For this review, take the finished solid that the model builds, in its own axes (mm). Face numbers are marked on the shaded views. A direction names the side the tool comes from. Coordinates: 2 decimals unless noted, no trailing zeros. Write each loop counter-clockwise with the first axis right and the second up, starting at its lowest first coordinate (ties: lowest second). Pieces come first, ordered by that corner, then holes. Notation, with made-up numbers: (88, -2.75) -> (105, -2.75) arc R19 cw to (105, 30.25) -> close; hole circle Ø4 at (-3, 24.5). An arc over 180 degrees is marked (long way). One line per item, written item: value. Start each with the question number.
1) Machinability: for the marked faces 4 and 5, which of the approach directions +Z, -Z, +X, -X, +Y, -Y give a long, thin tool a straight path to every point of the face, cutting with its end or side? Answer none if there is none.
2) Add section C-C (x = -0.6). State the section outline as (y, z) points, and give its area (3 significant figures).
3) Mouldability with a two-part tool opening along Z and no side actions: class the marked faces 1, 2 and 3 as released by +Z, released by -Z, zero draft, split by the parting line, or undercut.
4) Add section A-A (z = 0). State the section outline as (x, y) points, and give its area (3 significant figures).
5) For pin 1 Ø1.5 at (x, y) = (0, -2) entering from -Z; pin 2 Ø1 at (x, z) = (0.5, -2) entering from +Y; pin 3 Ø1.5 at (x, z) = (0, 1.5) entering from -Y, all flat-tipped, find the tip position at first contact; note any pin that passes through.
6) Add section D-D (x = 2.25). State the section outline as (y, z) points.
7) For probe 1 along Z at (x, y) = (0.2, 0); probe 2 along Z at (x, y) = (0.35, -0.65); probe 3 along X at (y, z) = (2.1, -0.2), list the stretches that pass through material, from the lowest coordinate up. Write a range as from..to.
from build123d import *

# Parameters (mm, degrees)
F0_R     = 2.85
F1_DEPTH = 3
F2_SIZE2 = 0.6
F2_SIZE  = 0.4
F3_R     = 1.45
F4_DEPTH = 2
F5_R     = 1.95
F5_R_2   = 1.45
F6_DEPTH = 0.5
F7_SIZE  = 0.2


with BuildPart() as f1:
    # F0 (on Right) → F1 (new body)
    with BuildSketch(Plane.YZ):
        Circle(F0_R)
    extrude(amount=F1_DEPTH)

    # F2
    f2_edges = [f1.edges().sort_by_distance(p)[0] for p in [
        (3, -2.85, 0),
    ]]
    f2_side = f1.faces().sort_by_distance((3, 0, 0))[0]
    chamfer(f2_edges, length=F2_SIZE, length2=F2_SIZE2, reference=f2_side)

    # F3 (on face) → F4 (join)
    with BuildSketch(Plane(origin=(0, 0, 0), x_dir=(0, -1, 0), z_dir=(-1, 0, 0))):
        Circle(F3_R)
    extrude(amount=F4_DEPTH)

    # F5 (on face) → F6 (cut)
    with BuildSketch(Plane(origin=(0, 0, 0), x_dir=(0, -1, 0), z_dir=(-1, 0, 0))):
        Circle(F5_R)
        Circle(F5_R_2, mode=Mode.SUBTRACT)
    extrude(amount=-F6_DEPTH, mode=Mode.SUBTRACT)

    # F7
    f7_edges = [f1.edges().sort_by_distance(p)[0] for p in [
        (0.5, 1.95, 0),
    ]]
    chamfer(f7_edges, length=F7_SIZE)


solid = f1.part
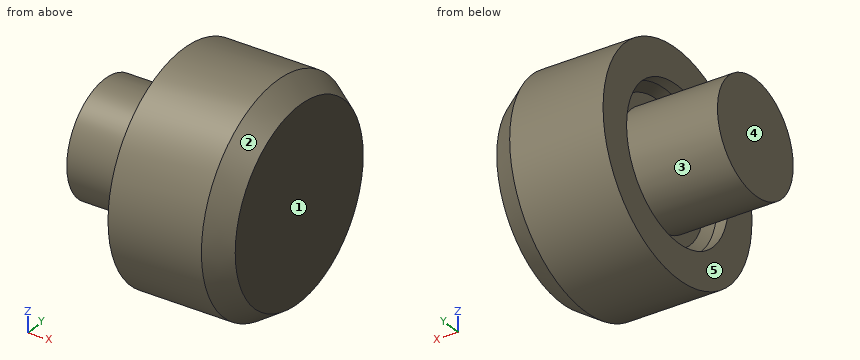
Numbers:
1. face 4: +Z, -Z, -X, +Y, -Y
1. face 5: -X
2. outline: circle Ø2.9 at (0, 0)
2. area: 6.61 mm²
3. face 1: zero draft
3. face 2: split by the parting line
3. face 3: undercut
4. outline: (-2, -1.45) -> (0.5, -1.45) -> (0.5, -1.75) -> (0.3, -1.95) -> (0, -1.95) -> (0, -2.85) -> (2.4, -2.85) -> (3, -2.45) -> (3, 2.45) -> (2.4, 2.85) -> (0, 2.85) -> (0, 1.95) -> (0.3, 1.95) -> (0.5, 1.75) -> (0.5, 1.45) -> (-2, 1.45) -> close
4. area: 22.2 mm²
5. pin 1: z = -2.56
5. pin 2: y = 2.42
5. pin 3: y = -2.75
6. outline: circle Ø5.7 at (0, 0)
7. probe 1: -2.85..-1.95, -1.45..1.45, 1.95..2.85
7. probe 2: -2.77..-1.79, -1.3..1.3, 1.79..2.77
7. probe 3: 0..3
